```python
from build123d import *

# Parameters (mm, degrees)
F1_R     = 3.175
F2_DEPTH = 15.875


with BuildPart() as f2:
    # F1 (on Right) → F2 (new body, symmetric)
    with BuildSketch(Plane.YZ):
        Circle(F1_R)
    extrude(amount=F2_DEPTH, both=True)

    # F0 (on Top) → F3 (revolve)
    with BuildSketch(Plane.XY):
        Polygon((-12.7, 0), (12.7, 0), (12.7, 1.5875), (9.525, 1.5875), (9.525, 9.8425), (6.35, 9.8425), (6.35, 3.175), (0, 3.175), (-6.35, 3.175), (-6.35, 9.8425), (-9.525, 9.8425), (-9.525, 1.5875), (-12.7, 1.5875), align=None)
    revolve(axis=Axis((0, 0, 0), (1, 0, 0)))


solid = f2.part
```
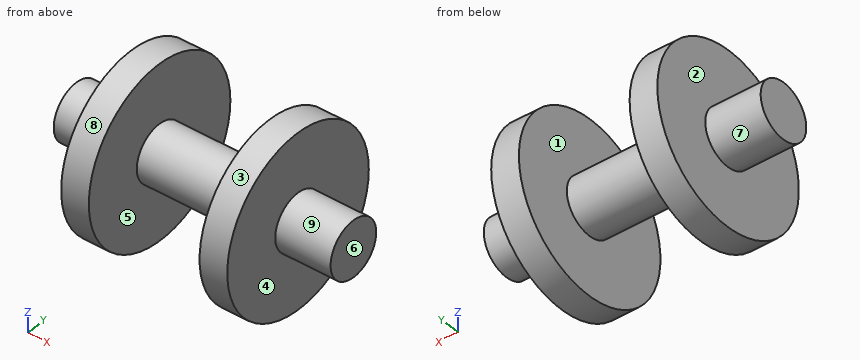
Geometry: final body of the model. Coordinates: model frame, mm. Face numbers are marked on the shaded views. A direction names the side the tool comes from. Coordinates: 2 decimals unless noted, no trailing zeros. Order: outer loops, then holes, each group sorted by start corner. A loop starts at its lowest first (then second) coordinate and runs counter-clockwise, first axis right, second up. Notation, with made-up numbers: (4, -32.75) - (41, -32.75) arc R31 ccw to (41, 4.25) - close; hole circle Ø5 at (36.25, 9). An arc over 180 degrees is marked (long way). Write each question's results on one line, items separated by ' | '.
1) Pull-direction query (X, two-part tool) for the marked faces 1, 2, 3 and 4; classes: pulls with the +X half, pulls with the -X half, needs draft (parallel to the pull), parting line crosses it, or undercut.
Results list:
face 1: undercut | face 2: pulls with the -X half | face 3: needs draft | face 4: pulls with the +X half
2) Section A-A, the plane y = -4.5. Return loops of the section in (x, z) (3 decimals), plus the area to 3 significant figures.
Results list:
outline: (-9.525, -8.754) - (-6.35, -8.754) - (-6.35, 8.754) - (-9.525, 8.754) - close; (6.35, -8.754) - (9.525, -8.754) - (9.525, 8.754) - (6.35, 8.754) - close | area: 111 mm^2
3) Section D-D, the plane z = 4. Return loops of the section in (x, y) (3 decimals), plus the area to 3 significant figures.
Results list:
outline: (-9.525, -8.993) - (-6.35, -8.993) - (-6.35, 8.993) - (-9.525, 8.993) - close; (6.35, -8.993) - (9.525, -8.993) - (9.525, 8.993) - (6.35, 8.993) - close | area: 114 mm^2
4) Set-up query: the marked faces 5, 6, 7, 8 and 9. Return all of +Z, -Z, +X, -X, +Y, -Y with unobstructed straight access to the full face (end or side cutting, diameter ignored); none if empty.
Results list:
face 5: none | face 6: +Z, -Z, +X, +Y, -Y | face 7: -X | face 8: +X, -X | face 9: +X
5) Pin query (flat end, axial travel): pin 1 (5 mm diameter, centred on x = -9.5, y = 2.5, fed in from +Z); pin 2 (2 mm diameter, centred on y = -5, z = -3.5, fed in from +X) (3 decimals); pin 3 (2 mm diameter, centred on x = 4.5, z = -2.5, fed in from -Y); pin 4 (6 mm diameter, centred on y = -7, z = -2, fed in from -X) (3 decimals). Return the tip coordinate at first contact, or that it passes through.
Results list:
pin 1: z = 9.84 | pin 2: x = 9.525 | pin 3: y = -2.8 | pin 4: x = -9.525
6) Line query: line 1 (X direction, y = -2.5, z = 4.5) (3 decimals); line 2 (Y direction, x = -7, z = -4.75); line 3 (Y direction, x = 8, z = 2.5). Output: solid intervals per line, ascending. Write a range as from..to.
Results list:
line 1: -9.525..-6.35, 6.35..9.525 | line 2: -8.62..8.62 | line 3: -9.52..9.52
